Check sheet for the modelled part. Datum: model origin and axes. Units: mm. Face numbers are marked on the shaded views. A direction names the side the tool comes from. Give positions to 0.01 mm unless a question says otherwise; leave off trailing zeros. Order: outer loops, then holes, each group sorted by start corner. A loop starts at its lowest first (then second) coordinate and runs counter-clockwise, first axis right, second up.
from build123d import *

# Parameters (mm, degrees)
CHANFRO1_SIZE         = 3.96875
CORTE_REVOLU_O1_ANGLE = 10
PADR_OCIRCULAR1_COUNT = 18
ESBO_O8_W             = 10
ESBO_O8_H             = 10
CORTE_EXTRUS_O1_DEPTH = 92.04375


with BuildPart() as part:
    # Esboço1 → Revolução1 (revolve)
    with BuildSketch(Plane.XY):
        Polygon((0, 20), (0, 39.6875), (26.19375, 39.6875), (26.19375, 91.44), (96.04375, 49.469885761), (96.04375, 20), align=None)
    revolve(axis=Axis((206.361590972, 0, 0), (-1, 0, 0)))

    # Chanfro1
    chanfro1_edges = [part.edges().sort_by_distance(p)[0] for p in [
        (0, -39.6875, 0),
    ]]
    chamfer(chanfro1_edges, length=CHANFRO1_SIZE)

    # Esboço3 → Corte-Revolução1 (revolve, symmetric, cut)
    with BuildSketch(Plane.XY) as corte_revolu_o1_sk:
        Polygon((96.04375, 49.469885761), (26.19375, 91.44), (26.19375, 81.455895118), (96.04375, 39.485780879), align=None)
    corte_revolu_o1 = revolve(axis=Axis((96.04375, 0, 0), (1, 0, 0)), revolution_arc=CORTE_REVOLU_O1_ANGLE / 2, mode=Mode.SUBTRACT)
    corte_revolu_o1 = corte_revolu_o1 + revolve(corte_revolu_o1_sk.sketch, axis=Axis((96.04375, 0, 0), (-1, 0, 0)), revolution_arc=CORTE_REVOLU_O1_ANGLE / 2, mode=Mode.SUBTRACT)

    # PadrãoCircular1: Corte-Revolução1 ×18 about axis
    padr_ocircular1_axis = Axis((0, 0, 0), (1, 0, 0))
    for i in range(1, PADR_OCIRCULAR1_COUNT):
        add(corte_revolu_o1.rotate(padr_ocircular1_axis, i * 360 / PADR_OCIRCULAR1_COUNT), mode=Mode.SUBTRACT)

    # Esboço7 → Corte-Revolução2 (revolve, cut)
    with BuildSketch(Plane(origin=(0, 0, 0), x_dir=(1, 0, 0), z_dir=(0, 1, 0)), mode=Mode.PRIVATE) as corte_revolu_o2_sk:
        Polygon((96.04375, 0), (96.04375, 49.28163791), (91.04375, 44.28163791), (91.04375, 0), align=None)
    revolve(corte_revolu_o2_sk.sketch.rotate(Axis((91.04375, 0, 0), (1, 0, 0)), 90), axis=Axis((91.04375, 0, 0), (1, 0, 0)), mode=Mode.SUBTRACT)  # turned: the seam where the file's is

    # Esboço8 → Corte-extrusão1 (cut, through all)
    with BuildSketch(Plane(origin=(91.04375, 0, 0), x_dir=(0, 0, -1), z_dir=(1, 0, 0))):
        with Locations((0, 20)):
            Rectangle(ESBO_O8_W, ESBO_O8_H)
    extrude(amount=-CORTE_EXTRUS_O1_DEPTH, mode=Mode.SUBTRACT)


solid = part.part
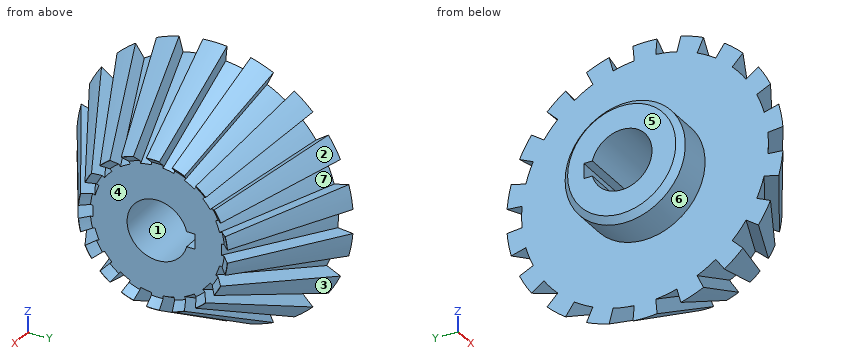
1) Section check C-C, the plane y = 60. State how many separate pieces and enclosed holes the cut face has, then the cut area to 3 significant figures.
Recorded:
separate pieces: 3
enclosed holes: 0
area: 3,470 mm2
2) Section check B-B, the plane z = 0. Record the cut outline in (x, y), then the cut area to 3 significant figures.
Recorded:
outline: (0, -35.72) - (3.97, -39.69) - (26.19, -39.69) - (26.19, -81.46) - (91.04, -42.49) - (91.04, -20) - (0, -20) - close; (0, 25) - (91.04, 25) - (91.04, 42.49) - (26.19, 81.46) - (26.19, 39.69) - (3.97, 39.69) - (0, 35.72) - close
area: 6,000 mm2
3) Material ranges on L1, parallel to Z at x = 24, y = 0; L2, parallel to X at y = 81.5, z = 14.5; L3, parallel to Y at x = 46.5, z = 43, recorded low to high.
Recorded:
L1: z = -39.69 to -20, 20 to 39.69
L2: x = 26.19 to 40.61
L3: y = -66.56 to -61.41, -54.29 to 54.29, 61.41 to 66.56
4) Section check A-A, the plane y = 0. Record the cut outline in (x, z), then the cut area to 3 significant figures.
Recorded:
outline: (0, -35.72) - (3.97, -39.69) - (26.19, -39.69) - (26.19, -91.44) - (96.04, -49.47) - (96.04, -49.28) - (91.04, -44.28) - (91.04, -20) - (0, -20) - close; (0, 20) - (91.04, 20) - (91.04, 44.28) - (96.04, 49.28) - (96.04, 49.47) - (26.19, 91.44) - (26.19, 39.69) - (3.97, 39.69) - (0, 35.72) - close
area: 7,800 mm2
5) Draft check along Z on the marked faces 1, 2, 3 and 4. Enter one of: +Z half, -Z half, draft (parallel to the pull), parting line (faces both ways), or undercut.
Recorded:
face 1: undercut
face 2: +Z half
face 3: -Z half
face 4: undercut
6) Set-up check for the marked faces 5, 6 and 7: record each of +Z, -Z, +X, -X, +Y, -Y from which the full face is reachable in a straight line by a thin tool's end or side.
Recorded:
face 5: +Z, -Z, -X, +Y, -Y
face 6: -X
face 7: +X
7) Depth check by flat-ended pin: pin 1 Ø3 at (x, y) = (37.5, -46.5) entering from -Z; pin 2 Ø3 at (x, z) = (39, -0.5) entering from -Y; pin 3 Ø6 at (x, z) = (79.5, 3) entering from +Y. Enter the tip coordinate at first touch or a pass-through.
Recorded:
pin 1: stops at z = -68.55
pin 2: stops at y = -74.66
pin 3: stops at y = 60.35
